```python
from build123d import *

# Parameters (mm, degrees)
SKETCH1_W           = 60
SKETCH1_H           = 65
BOSS_EXTRUDE1_DEPTH = 10
SKETCH6_W           = 60
SKETCH6_H           = 10
BOSS_EXTRUDE2_DEPTH = 23
CHAMFER1_SIZE       = 5
CHAMFER1_SIZE2      = 2.886751346
SKETCH5_R           = 11
CUT_EXTRUDE4_DEPTH  = 7
SKETCH12_R          = 2.5
CUT_EXTRUDE6_DEPTH  = 108.953693777
RIB1_REACH          = 81.712
SKETCH13_WALL_W     = 178.916818752
SKETCH13_WALL_H     = 10
CHAMFER3_START      = -1
CHAMFER3_DEPTH      = 24
SKETCH14_R          = 1.175
SKETCH14_R_2        = 1.25
CUT_EXTRUDE7_DEPTH  = 5


with BuildPart() as part:
    # Sketch1 → Boss-Extrude1 (new body)
    with BuildSketch(Plane.XY):
        with Locations((60, 32.5)):
            Rectangle(SKETCH1_W, SKETCH1_H)
    extrude(amount=BOSS_EXTRUDE1_DEPTH)

    # Sketch6 → Boss-Extrude2 (add)
    with BuildSketch(Plane(origin=(0, 0, 0), x_dir=(-1, 0, 0), z_dir=(0, 0, -1))):
        with Locations((-60, 60)):
            Rectangle(SKETCH6_W, SKETCH6_H)
    extrude(amount=-BOSS_EXTRUDE2_DEPTH)

    # Chamfer1
    chamfer1_edges = [part.edges().sort_by_distance(p)[0] for p in [
        (60, 65, 0),
        (90, 32.5, 0),
        (60, 0, 0),
        (30, 32.5, 0),
    ]]
    chamfer1_side = [part.faces().sort_by_distance(p)[0] for p in [
        (60, 32.5, 0),
    ]]
    chamfer(chamfer1_edges, length=CHAMFER1_SIZE, length2=CHAMFER1_SIZE2, reference=chamfer1_side[0])

    # Sketch5 → Cut-Extrude4 (cut)
    with BuildSketch(Plane.XY.offset(10)):
        with Locations((60, 17.17)):
            Circle(SKETCH5_R)
    extrude(amount=-CUT_EXTRUDE4_DEPTH, mode=Mode.SUBTRACT)

    # Sketch12 → Cut-Extrude6 (cut, through all)
    with BuildSketch(Plane(origin=(0, 55, 0), x_dir=(-1, 0, 0), z_dir=(0, -1, 0))):
        with Locations(Location((-80, -17, 0), (0, 0, 180))):
            Circle(SKETCH12_R)
        with Locations((-40, -17)):
            Circle(SKETCH12_R)
    extrude(amount=-CUT_EXTRUDE6_DEPTH, mode=Mode.SUBTRACT)

    # Sketch13 wall → Rib1 (add, up to next)
    with BuildSketch(Plane(origin=(50, 47.5, 14.5), x_dir=(0, -0.857492925713, -0.514495755428), z_dir=(0, 0.514495755428, -0.857492925713)), mode=Mode.PRIVATE) as rib1_sk1:
        Rectangle(SKETCH13_WALL_W, SKETCH13_WALL_H)
    rib1_tool1 = extrude(rib1_sk1.sketch, amount=RIB1_REACH, mode=Mode.PRIVATE) - part.part
    rib1 = rib1_tool1.solids().sort_by_distance((50, 47.5, 14.5))[0]
    add(rib1)

    # Mirror1: Rib1 across plane
    add(rib1.mirror(Plane(origin=(60, 0, 0), x_dir=(0, 0, 1), z_dir=(1, 0, 0))))

    # Chamfer3: read off the stored shape, not the designer's step
    # Chamfer3 outline → Chamfer3 (cut)
    with BuildSketch(Plane.XY.offset(CHAMFER3_START)):
        Polygon((90, 0), (90, 10), (80, 0), align=None)
        Polygon((30, 0), (40, 0), (30, 10), align=None)
    extrude(amount=CHAMFER3_DEPTH, mode=Mode.SUBTRACT)

    # Sketch14 → Cut-Extrude7 (cut)
    with BuildSketch(Plane.ZY.offset(-30)):
        with Locations((7.3, 24.6)):
            Circle(SKETCH14_R)
        with Locations((7.3, 15.1)):
            Circle(SKETCH14_R_2)
    extrude(amount=-CUT_EXTRUDE7_DEPTH, mode=Mode.SUBTRACT)


solid = part.part
```
Read the model definition and answer for the solid it produces. Units are mm, in the model's axes. A direction names the side the tool comes from. Coordinates: 2 decimals unless noted, no trailing zeros. Loops run counter-clockwise (first coordinate to the right, second up) from the corner with the lowest first, then second, coordinate; pieces in that order, holes last. Notation, with made-up numbers: (4, 52.5) - (21, 52.5) arc R28 ccw to (21, 85.5) - close; hole circle Ø5 at (45, 17). An arc over 180 degrees is marked (long way). Answer in a Markdown table with one row per item.
1. Find section A-A, the plane z = 7.3. Write down the section's boundary in (x, y) (3 decimals), then the cut area to 3 significant figures.
Conclusion:
| item | result |
|---|---|
| outline | (30, 10) - (40, 0) - (80, 0) - (90, 10) - (90, 65) - (30, 65) - (30, 25.775) - (35, 25.775) - (35, 23.425) - (30, 23.425) - (30, 16.35) - (35, 16.35) - (35, 13.85) - (30, 13.85) - close; hole circle Ø22 at (60, 17.17) |
| area | 3,400 mm² |
2. Given pin 1 (4.5 mm diameter, centred on y = 49.5, z = 13, fed in from -X); pin 2 (1.5 mm diameter, centred on x = 38, y = 7.5, fed in from +Z); pin 3 (8 mm diameter, centred on x = 65, y = 46.5, fed in from +Z); pin 4 (3 mm diameter, centred on x = 80, z = 17, fed in from +Y), each flat-ended and moving along its own axis, determine where each tip first touches the part or whether it passes through.
Conclusion:
| item | result |
|---|---|
| pin 1 | stops at x = 45 |
| pin 2 | stops at z = 10 |
| pin 3 | stops at z = 16.3 |
| pin 4 | passes through |
3. Find section D-D, the plane z = 17. Write down the section's boundary in (x, y).
Conclusion:
| item | result |
|---|---|
| outline | (30, 55) - (37.5, 55) - (37.5, 65) - (30, 65) - close; (42.5, 55) - (45, 55) - (45, 51.67) - (55, 51.67) - (55, 55) - (65, 55) - (65, 51.67) - (75, 51.67) - (75, 55) - (77.5, 55) - (77.5, 65) - (42.5, 65) - close; (82.5, 55) - (90, 55) - (90, 65) - (82.5, 65) - close |
4. Straight lines are drawn through the part: line 1 (Y direction, x = 31.4, z = 7.3) (3 decimals); line 2 (Y direction, x = 32.5, z = 7.3) (3 decimals); line 3 (Y direction, x = 60, z = 6.25). For each, find the intervals that lie inside material, in ascending order.
Conclusion:
| item | result |
|---|---|
| line 1 | y = 8.6 to 13.85, 16.35 to 23.425, 25.775 to 65 |
| line 2 | y = 7.5 to 13.85, 16.35 to 23.425, 25.775 to 65 |
| line 3 | y = 0 to 6.17, 28.17 to 65 |
5. Find section B-B, the plane x = 60. Write down the section's boundary in (y, z), then the cut area to 3 significant figures.
Conclusion:
| item | result |
|---|---|
| outline | (0, 2.89) - (5, 0) - (60, 0) - (65, 2.89) - (65, 23) - (55, 23) - (55, 10) - (28.17, 10) - (28.17, 3) - (6.17, 3) - (6.17, 10) - (0, 10) - close |
| area | 612 mm² |
6. Determine the mould class of faces 4 (the face through (60, 55, 18)), 5 (the face through (49.01, 17.65, 6.55)), 6 (the face through (60, 17, 3)), 7 (the face through (77.5, 59.9, 17.1)) for opening direction Y: +Y half, -Y half, draft (parallel to the pull), parting line (faces both ways), or undercut.
Conclusion:
| item | result |
|---|---|
| face 4 | -Y half |
| face 5 | undercut |
| face 6 | undercut |
| face 7 | draft |
7. Which of the six approach directions +Z, -Z, +X, -X, +Y, -Y give full straight-line access (tool end or side, diameter ignored) to faces 1 (the face through (32.465, 23.558, 7.842)), 2 (the face through (49.93, 47.605, 14.563)), 3 (the face through (55, 51, 13))?
Conclusion:
| item | result |
|---|---|
| face 1 | -X |
| face 2 | +Z, +X, -X, -Y |
| face 3 | +Z, -Y |
8. Find section C-C, the plane y = 17.17. Write down the section's boundary in (x, z).
Conclusion:
| item | result |
|---|---|
| outline | (30, 2.89) - (35, 0) - (85, 0) - (90, 2.89) - (90, 10) - (71, 10) - (71, 3) - (49, 3) - (49, 10) - (30, 10) - close |
